from build123d import *

# Parameters (mm, degrees)
SKETCH1_W           = 6.35
SKETCH1_H           = 120.65
EXTRUDE_THIN1_DEPTH = 4.572
SKETCH2_R           = 1.651
CUT_EXTRUDE1_DEPTH  = 4.572
LPATTERN1_COUNT     = 6
LPATTERN1_PITCH     = 114.3
FILLET1_R           = 2.54


with BuildPart() as part:
    # Sketch1 → Extrude-Thin1 (new body)
    with BuildSketch(Plane(origin=(0, 0, 0), x_dir=(1, 0, 0), z_dir=(0, 1, 0))):
        with Locations((-3.175, -29.775350058)):
            Rectangle(SKETCH1_W, SKETCH1_H)
    extrude(amount=EXTRUDE_THIN1_DEPTH)

    # Sketch2 → Cut-Extrude1 (cut)
    with BuildSketch(Plane(origin=(0, 4.572, 0), x_dir=(1, 0, 0), z_dir=(0, 1, 0))):
        with Locations((-3.175, 27.432)):
            Circle(SKETCH2_R)
    cut_extrude1 = extrude(amount=-CUT_EXTRUDE1_DEPTH, mode=Mode.SUBTRACT)

    # LPattern1: Cut-Extrude1 ×6
    with Locations(*[(0, 0, i * LPATTERN1_PITCH) for i in range(1, LPATTERN1_COUNT)]):
        add(cut_extrude1, mode=Mode.SUBTRACT)

    # Fillet1
    fillet1_edges = [part.edges().sort_by_distance(p)[0] for p in [
        (-6.35, 2.286, -30.549649942),
        (0, 2.286, -30.549649942),
        (0, 2.286, 90.100350058),
        (-6.35, 2.286, 90.100350058),
    ]]
    fillet(fillet1_edges, radius=FILLET1_R)


solid = part.part
Could you check a few things on this model? Use its own coordinates, in mm. Coordinates: 2 decimals unless noted, no trailing zeros. Order: outer loops, then holes, each group sorted by start corner. A loop starts at its lowest first (then second) coordinate and runs counter-clockwise, first axis right, second up. Notation, with made-up numbers: (61, 85) - (72, 85) arc R10 ccw to (72, 99) - close; hole circle Ø5 at (46.5, 41). An arc over 180 degrees is marked (long way). Answer in a Markdown table with one row per item. Add a question column.
(1) I need wall thicknesses on L1, parallel to Z at x = -4.5, y = 2.5; L2, parallel to Z at x = -3.75, y = 2.1; L3, parallel to Z at x = -1, y = 1.85. Which ranges of each line are inside material? Lowest first, please.
(2) If we mould it in two halves opening along Z, with no side actions, what happens to faces 1 (the face through (-2.41, 2.32, 88.33)), 2 (the face through (-0.764, 2.318, 89.376)), 3 (the face through (-0.764, 2.318, -29.825))? For each: released by +Z, released by -Z, zero draft, split by the parting line, or undercut.
(3) If we section it at A-A, the plane y = 0.8: Please give me the cut outline in (x, z) (3 decimals), then the cut area to 3 significant figures.
Results are:
| question | item | result |
|---|---|---|
| 1 | L1 | z = -30.45 to -28.42, -26.45 to 85.88, 87.85 to 90 |
| 1 | L2 | z = -30.55 to -28.98, -25.88 to 85.32, 88.42 to 90.1 |
| 1 | L3 | z = -30.03 to 89.58 |
| 2 | face 1 | undercut |
| 2 | face 2 | released by +Z |
| 2 | face 3 | released by -Z |
| 3 | outline | (-6.35, -28.01) arc R2.54 ccw to (-3.81, -30.55) - (-2.54, -30.55) arc R2.54 ccw to (0, -28.01) - (0, 87.56) arc R2.54 ccw to (-2.54, 90.1) - (-3.81, 90.1) arc R2.54 ccw to (-6.35, 87.56) - close; hole circle Ø3.302 at (-3.175, -27.432); hole circle Ø3.302 at (-3.175, 86.868) |
| 3 | area | 743 mm2 |
